Here's how the part is built. I have some questions about the finished solid (model axes, mm). Round coordinates to 2 decimals unless told otherwise and drop trailing zeros. Write each loop counter-clockwise with the first axis right and the second up, starting at its lowest first coordinate (ties: lowest second). Pieces come first, ordered by that corner, then holes. Notation, with made-up numbers: (11, 85) - (51, 85) arc R13 ccw to (51, 104) - close; hole circle Ø9 at (68.5, -4). An arc over 180 degrees is marked (long way). Return JSON: item names as keys, results as strings. Group by question number.
```python
from build123d import *

# Parameters (mm, degrees)
F0_R     = 1.5875
F1_DEPTH = 12.7


with BuildPart() as f1:
    # F0 (on Top) → F1 (new body)
    with BuildSketch(Plane.XY):
        with BuildLine():
            ThreePointArc((4.517e-07, -333.375), (117.8658617487, -284.5533614293), (166.6875, -166.6875))
            Line((166.6875, -166.6875), (153.9875, -166.6875))
            ThreePointArc((153.9875, -166.6875), (0, -320.675), (-153.9875, -166.6875))
            Line((-153.9875, -166.6875), (-166.6875, -166.6875))
            ThreePointArc((-166.6875, -166.6875), (-117.8658614293, -284.5533617487), (4.517e-07, -333.375))
        make_face()
        with BuildLine():
            Line((153.9875, 166.6875), (166.6875, 166.6875))
            ThreePointArc((166.6875, 166.6875), (117.8658618859, 284.5533612921), (8.398e-07, 333.375))
            ThreePointArc((8.398e-07, 333.375), (-117.8658612921, 284.5533618859), (-166.6875, 166.6875))
            Line((-166.6875, 166.6875), (-153.9875, 166.6875))
            ThreePointArc((-153.9875, 166.6875), (0, 320.675), (153.9875, 166.6875))
        make_face()
        with BuildLine():
            ThreePointArc((-166.6875, -166.6875), (-117.865861589, -48.821638411), (0, 0))
            ThreePointArc((0, 0), (-117.865861589, 48.821638411), (-166.6875, 166.6875))
            Line((-166.6875, 166.6875), (-166.6875, -166.6875))
        make_face()
        with BuildLine():
            Line((153.9875, -166.6875), (166.6875, -166.6875))
            ThreePointArc((166.6875, -166.6875), (117.865861589, -48.821638411), (0, 0))
            Line((0, 0), (0, -4.7625))
            ThreePointArc((0, -4.7625), (1.1225320151, -5.2274679849), (1.5875, -6.35))
            ThreePointArc((1.5875, -6.35), (1.1225320151, -7.4725320151), (0, -7.9375))
            Line((0, -7.9375), (0, -12.7))
            ThreePointArc((0, -12.7), (108.885605468, -57.801894532), (153.9875, -166.6875))
        make_face()
        with BuildLine():
            ThreePointArc((0, 0), (117.865861589, 48.821638411), (166.6875, 166.6875))
            Line((166.6875, 166.6875), (153.9875, 166.6875))
            ThreePointArc((153.9875, 166.6875), (0, 12.7), (-153.9875, 166.6875))
            Line((-153.9875, 166.6875), (-166.6875, 166.6875))
            ThreePointArc((-166.6875, 166.6875), (-117.865861589, 48.821638411), (0, 0))
        make_face()
        with Locations((0, 6.35)):
            Circle(F0_R, mode=Mode.SUBTRACT)
        with BuildLine():
            ThreePointArc((0, 0), (117.865861589, -48.821638411), (166.6875, -166.6875))
            Line((166.6875, -166.6875), (166.6875, 166.6875))
            ThreePointArc((166.6875, 166.6875), (117.865861589, 48.821638411), (0, 0))
        make_face()
        with BuildLine():
            Line((-166.6875, -333.375), (4.517e-07, -333.375))
            ThreePointArc((4.517e-07, -333.375), (-117.8658614293, -284.5533617487), (-166.6875, -166.6875))
            Line((-166.6875, -166.6875), (-166.6875, -333.375))
        make_face()
        with BuildLine():
            Line((166.6875, -333.375), (166.6875, -166.6875))
            ThreePointArc((166.6875, -166.6875), (117.8658617487, -284.5533614293), (4.517e-07, -333.375))
            Line((4.517e-07, -333.375), (166.6875, -333.375))
        make_face()
        with BuildLine():
            ThreePointArc((-166.6875, 166.6875), (-117.8658612921, 284.5533618859), (8.398e-07, 333.375))
            Line((8.398e-07, 333.375), (-166.6875, 333.375))
            Line((-166.6875, 333.375), (-166.6875, 166.6875))
        make_face()
        with BuildLine():
            ThreePointArc((8.398e-07, 333.375), (117.8658618859, 284.5533612921), (166.6875, 166.6875))
            Line((166.6875, 166.6875), (166.6875, 333.375))
            Line((166.6875, 333.375), (8.398e-07, 333.375))
        make_face()
        with BuildLine():
            Line((0, -4.7625), (0, 0))
            ThreePointArc((0, 0), (-117.865861589, -48.821638411), (-166.6875, -166.6875))
            Line((-166.6875, -166.6875), (-153.9875, -166.6875))
            ThreePointArc((-153.9875, -166.6875), (-108.885605468, -57.801894532), (0, -12.7))
            Line((0, -12.7), (0, -7.9375))
            ThreePointArc((0, -7.9375), (-1.5875, -6.35), (0, -4.7625))
        make_face()
    extrude(amount=F1_DEPTH)


solid = f1.part
```
1) Imagine slicing it at B-B (y = -270.5). Please give me the cut outline in (x, z), plus the area to 3 significant figures.
2) I need wall thicknesses on line 1 along Y through (x, z) = (-3, 4.25) (3 decimals); line 2 along Y through (x, z) = (-71, 11) (3 decimals); line 3 along X through (y, z) = (162, 3). Which ranges of each line are inside material? Lowest first, please.
3) If we mould it in two halves opening along X, with no side actions, what happens to faces 1 (the cylindrical face through (146.877, 120.434, 6.261)), 2 (the flat face through (-166.688, 5, 6)), 3 (the cylindrical face through (-93.699, -288.887, 6.261)), 4 (the flat face through (2, 333.375, 6))? For each: released by +X, released by -X, zero draft, split by the parting line, or undercut.
4) Imagine slicing it at A-A (z = 10). Give the number of separate pieces and of enclosed holes in the cut face, plus the area to 3 significant figures.
5) Imagine slicing it at D-D (y = 278). Please give me the cut outline in (x, z), plus the area to 3 significant figures.
6) Imagine slicing it at C-C (x = -33.5). Please give me the cut outline in (y, z) (3 decimals).
Results found:
{
 "1": {"outline": "(-166.69, 0) - (-113.73, 0) - (-113.73, 12.7) - (-166.69, 12.7) - close; (113.73, 0) - (166.69, 0) - (166.69, 12.7) - (113.73, 12.7) - close", "area": "1,350 mm²"},
 "2": {"line 1": "y = -333.375 to -320.646, -12.729 to 12.729, 320.646 to 333.375", "line 2": "y = -333.375 to -303.33, -30.045 to 30.045, 303.33 to 333.375", "line 3": "x = -166.69 to -153.92, 153.92 to 166.69"},
 "3": {"face 1": "undercut", "face 2": "released by -X", "face 3": "undercut", "face 4": "zero draft"},
 "4": {"separate pieces": "1", "enclosed holes": "4", "area": "73,300 mm²"},
 "5": {"outline": "(-166.69, 0) - (-106.4, 0) - (-106.4, 12.7) - (-166.69, 12.7) - close; (106.4, 0) - (166.69, 0) - (166.69, 12.7) - (106.4, 12.7) - close", "area": "1,530 mm²"},
 "6": {"outline": "(-333.375, 0) - (-316.987, 0) - (-316.987, 12.7) - (-333.375, 12.7) - close; (-16.388, 0) - (16.388, 0) - (16.388, 12.7) - (-16.388, 12.7) - close; (316.987, 0) - (333.375, 0) - (333.375, 12.7) - (316.987, 12.7) - close"}
}
